Verification items for this drawing (mm, ordinates from the low corner). Round coordinates to 2 decimals unless told otherwise and drop trailing zeros. Order: outer loops, then holes, each group sorted by start corner. A loop starts at its lowest first (then second) coordinate and runs counter-clockwise, first axis right, second up.
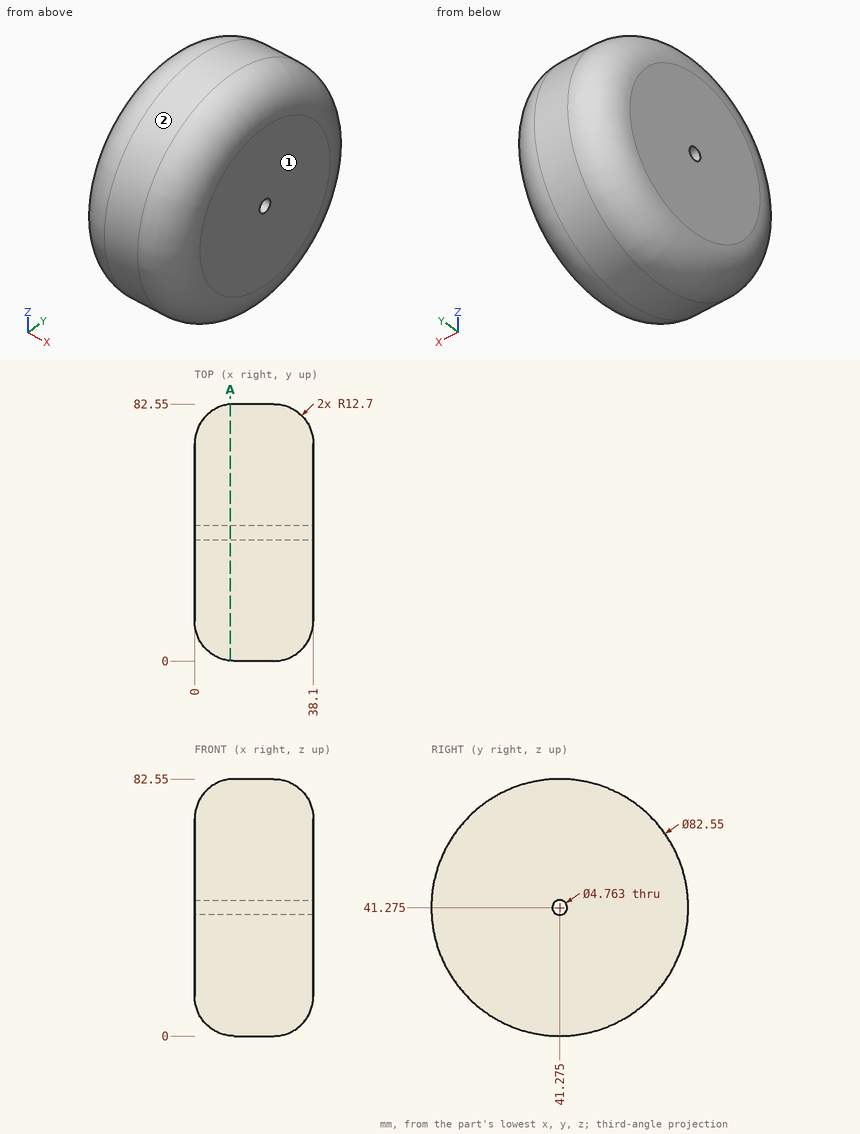
Item 1: Go/stop test with flat-tipped pins: P1, Ø2, axis at x = 12.5, y = 53, coming from the -Z side; P2, Ø5, axis at x = 15.5, y = 9, coming from the -Z side; P3, Ø10, axis at x = 21.5, y = 33, coming from the -Z side. Record where each tip stops, or that it passes through.
Answer:
P1: stops at z = 1.42
P2: stops at z = 12.69
P3: stops at z = 0.13
Item 2: Release check for a two-part mould opening along Z. For the marked faces 1 and 2 record: released by +Z, released by -Z, zero draft, split by the parting line, or undercut.
Answer:
face 1: zero draft
face 2: split by the parting line
Item 3: Sectioned sample at A-A (x = 11.5). Record the cut outline in (y, z) (1 decimal), and give its area (3 significant figures).
Answer:
outline: circle Ø82.4 at (41.3, 41.3); hole circle Ø4.8 at (41.3, 41.3)
area: 5,320 mm2
Item 4: Scan lines: line 1 along Y through (x, z) = (18, 41); line 2 along Y through (x, z) = (15, 22); line 3 along Z through (x, y) = (4.5, 53) (1 decimal). Record each from-to range of solid material in increasing order.
Answer:
line 1: y = 0 to 38.91, 43.64 to 82.55
line 2: y = 4.78 to 77.77
line 3: z = 4.8 to 77.7
